The model under review builds one solid part; all positions refer to its coordinate system, in mm. A direction names the side the tool comes from. Coordinates: 2 decimals unless noted, no trailing zeros. Loops run counter-clockwise (first coordinate to the right, second up) from the corner with the lowest first, then second, coordinate; pieces in that order, holes last. Notation, with made-up numbers: (6, -22) - (49, -22) arc R21 ccw to (49, 13) - close; hole circle Ø5 at (-9.5, 38). An arc over 180 degrees is marked (long way). Use a Markdown table: item, result. Add a question column.
1) Clearance check with flat-ended pins moving along their axes: pin 1 (1.3 mm diameter, centred on y = 43, z = 2, fed in from -X); pin 2 (0.8 mm diameter, centred on y = 48, z = 1, fed in from +X); pin 3 (1.3 mm diameter, centred on x = 49.5, z = 2, fed in from +Y); pin 4 (6 mm diameter, centred on x = 51, y = 70.5, fed in from -Z). State where each tip first meets the part, or that it passes through.
2) For faces 1 (the flat face through (1.12, 82, 1)), 2 (the flat face through (48, 87.118, 1)), 3 (the flat face through (6, 33.918, 1)), 4 (the flat face through (48, 12.318, 1)), 5 (the flat face through (91, 33.918, 1)), list the 3-axis set-ups (+Z, -Z, +X, -X, +Y, -Y) from which the entire face can be reached by the end or side of a thin tool; tool diameter is ignored.
3) Add section B-B, the plane z = 0.5. Give the boundary of the cut face in (x, y), and give its area (3 significant figures).
4) The part is to be moulded in two halves that separate along X. For faces 6 (the flat face through (32.72, 7, 1)), 7 (the flat face through (91, 65.518, 1)), 8 (the flat face through (85.92, 49, 1)), say which applies: pulls with the +X half, pulls with the -X half, needs draft (parallel to the pull), parting line crosses it, or undercut.
5) Add section A-A, the plane y = 8.5. Give the boundary of the cut face in (x, z).
6) To check wall thickness, follow L1, parallel to Y at x = 87.5, z = 1.5; L2, parallel to X at y = 10, z = 0.45; L3, parallel to X at y = 37.5, z = 0.7. State the ranges of each line that lie inside material, in increasing order. Write a range as [from, to].
7) Add section C-C, the plane y = 59. Give the boundary of the cut face in (x, z), and give its area (3 significant figures).
8) Add section D-D, the plane x = 35.5. Give the boundary of the cut face in (y, z).
```python
from build123d import *

# Parameters (mm, degrees)
BOSS_EXTRUDE1_DEPTH = 2.6
SKETCH2_W           = 10
SKETCH2_H           = 31.6
SKETCH2_W_2         = 31.6
SKETCH2_H_2         = 10
CUT_EXTRUDE1_DEPTH  = 3.6


with BuildPart() as part:
    # Sketch1 → Boss-Extrude1 (new body)
    with BuildSketch(Plane.XY):
        Polygon((1.120381921, 67.197647161), (1.120381921, 32.237647161), (1.120381921, 2.317647161), (31.040381921, 2.317647161), (66.000381921, 2.317647161), (95.920381921, 2.317647161), (95.920381921, 32.237647161), (95.920381921, 62.157647161), (95.920381921, 97.117647161), (60.960381921, 97.117647161), (31.040381921, 97.117647161), (1.120381921, 97.117647161), align=None)
    extrude(amount=BOSS_EXTRUDE1_DEPTH)

    # Sketch2 → Cut-Extrude1 (cut, through all)
    with BuildSketch(Plane.XY.offset(2.6)):
        with Locations((6.120381921, 49.717647161)):
            Rectangle(SKETCH2_W, SKETCH2_H)
        with Locations((90.920381921, 49.717647161)):
            Rectangle(SKETCH2_W, SKETCH2_H)
        with Locations((48.520381921, 92.117647161)):
            Rectangle(SKETCH2_W_2, SKETCH2_H_2)
        with Locations((48.520381921, 7.317647161)):
            Rectangle(SKETCH2_W_2, SKETCH2_H_2)
    extrude(amount=-CUT_EXTRUDE1_DEPTH, mode=Mode.SUBTRACT)


solid = part.part
```
From the geometry:
| question | item | result |
|---|---|---|
| 1 | pin 1 | stops at x = 11.12 |
| 1 | pin 2 | stops at x = 85.92 |
| 1 | pin 3 | stops at y = 87.12 |
| 1 | pin 4 | stops at z = 0 |
| 2 | face 1 | +Z, -Z, -X, +Y, -Y |
| 2 | face 2 | +Z, -Z, +Y |
| 2 | face 3 | +Z, -Z, -X |
| 2 | face 4 | +Z, -Z, -Y |
| 2 | face 5 | +Z, -Z, +X |
| 3 | outline | (1.12, 2.32) - (32.72, 2.32) - (32.72, 12.32) - (64.32, 12.32) - (64.32, 2.32) - (95.92, 2.32) - (95.92, 33.92) - (85.92, 33.92) - (85.92, 65.52) - (95.92, 65.52) - (95.92, 97.12) - (64.32, 97.12) - (64.32, 87.12) - (32.72, 87.12) - (32.72, 97.12) - (1.12, 97.12) - (1.12, 65.52) - (11.12, 65.52) - (11.12, 33.92) - (1.12, 33.92) - close |
| 3 | area | 7,720 mm^2 |
| 4 | face 6 | undercut |
| 4 | face 7 | needs draft |
| 4 | face 8 | pulls with the +X half |
| 5 | outline | (1.12, 0) - (32.72, 0) - (32.72, 2.6) - (1.12, 2.6) - close; (64.32, 0) - (95.92, 0) - (95.92, 2.6) - (64.32, 2.6) - close |
| 6 | L1 | y = [2.32, 33.92], [65.52, 97.12] |
| 6 | L2 | x = [1.12, 32.72], [64.32, 95.92] |
| 6 | L3 | x = [11.12, 85.92] |
| 7 | outline | (11.12, 0) - (85.92, 0) - (85.92, 2.6) - (11.12, 2.6) - close |
| 7 | area | 194 mm^2 |
| 8 | outline | (12.32, 0) - (87.12, 0) - (87.12, 2.6) - (12.32, 2.6) - close |
